Build history of the part. All positions in model axes, mm. A direction names the side the tool comes from. Give positions to 0.01 mm unless a question says otherwise; leave off trailing zeros. Loops run counter-clockwise (first coordinate to the right, second up) from the corner with the lowest first, then second, coordinate; pieces in that order, holes last. Notation, with made-up numbers: (-18, 38.25) -> (28, 38.25) arc R18 ccw to (28, 53.25) -> close; hole circle Ø1 at (43, -28.5). An arc over 180 degrees is marked (long way). Answer as a JSON object with one key per item and string values. Group by question number.
Q1. Band-saw the part on A-A, the plane x = 0. Write the cut outline in (y, z).
Q2. Band-saw the part on B-B, the plane y = 64.5. Write the cut outline in (x, z), plus the area to 3 significant figures.
Q3. Two-plate mould, pull along X, no slides. Class faces 4 (the flat face through (0, 96, -48.1)), 5 (the flat face through (-23, 0, 0)), 6 (the flat face through (21, 77.2, 5)): pulls with the +X half, pulls with the -X half, needs draft (parallel to the pull), parting line crosses it, or undercut.
Q4. Band-saw the part on C-C, the plane y = 0. Write the cut outline in (x, z), plus the area to 3 significant figures.
Q5. Tool access for faces 1 (the cylindrical face through (28.366, -3.312, -3.612)), 2 (the flat face through (28.762, 66, 4)), 3 (the flat face through (-6, 119.7, -2)): list every direction of +Z, -Z, +X, -X, +Y, -Y with a clear straight run to the whole face (end or side of a thin tool).
Q6. Band-saw the part on D-D, the plane z = -22.5. Write the cut outline in (x, y), plus the area to 3 significant figures.
Q7. Wall check: probe 1 along Y at (x, z) = (-15.5, -14); probe 2 along Y at (x, z) = (3, -12); probe 3 along Z at (x, y) = (4.5, 85.5). Give the ranges that are in metal, low to high. Write a range as from..to.
Q8. Drop flat-ended pins along their axis: pin 1 (17.5 mm diameter, centred on y = 27, z = 7, fed in from +X); pin 2 (1.4 mm diameter, centred on x = 27, y = 92.5, fed in from -Z); pin 3 (4 mm diameter, centred on x = 21.5, z = 10.5, fed in from +Y). Give the stop position or say it passes through.
from build123d import *

# Parameters (mm, degrees)
SKETCH1_W                 = 46
SKETCH1_H                 = 40.2
BOSS_EXTRUDE1_DEPTH       = 65.1
SKETCH3_R                 = 14
BOSS_EXTRUDE2_DEPTH       = 3
SKETCH4_R                 = 4.9
BOSS_EXTRUDE3_DEPTH       = 4.8
SKETCH7_W                 = 40.2
SKETCH7_H                 = 35.4
BOSS_EXTRUDE6_DEPTH       = 1
CHAMFER1_SIZE             = 6
CHAMFER1_SIZE2            = 5.1
MIRROR3_START             = 44.200099823
MIRROR3_OUTLINE_W         = 50
MIRROR3_OUTLINE_H         = 11
MIRROR3_DEPTH             = 3.885890521
CHAMFER1_OF_MIRROR8_SIZE2 = 5.1
CHAMFER1_OF_MIRROR8_SIZE  = 6
BOSS_EXTRUDE7_DEPTH       = 4.7625
SKETCH9_W                 = 40.2
SKETCH9_H                 = 61.1
BOSS_EXTRUDE8_DEPTH       = 41
SKETCH10_W                = 38
SKETCH10_H                = 38
BOSS_EXTRUDE9_DEPTH       = 9.3
SKETCH11_R                = 14
BOSS_EXTRUDE10_DEPTH      = 3
SKETCH12_R                = 4.9
BOSS_EXTRUDE11_DEPTH      = 4.8


# Read off the part's stored shape, not the designer's step: Mirror3
with BuildPart() as part:
    # Sketch1 → Boss-Extrude1 (new body)
    with BuildSketch(Plane(origin=(0, -14.5, 0), x_dir=(-1, 0, 0), z_dir=(0, 1, 0))):
        Rectangle(SKETCH1_W, SKETCH1_H)
    extrude(amount=BOSS_EXTRUDE1_DEPTH)

    # Sketch3 → Boss-Extrude2 (add)
    with BuildSketch(Plane.ZY.offset(-23)):
        Circle(SKETCH3_R)
    extrude(amount=-BOSS_EXTRUDE2_DEPTH)

    # Sketch4 → Boss-Extrude3 (add)
    with BuildSketch(Plane(origin=(26, 0, 0), x_dir=(0, 0, -1), z_dir=(1, 0, 0))):
        with Locations(Location((0, 0, 0), (0, 0, 180))):
            Circle(SKETCH4_R)
    extrude(amount=BOSS_EXTRUDE3_DEPTH)

    # Sketch7 → Boss-Extrude6 (add)
    with BuildSketch(Plane.ZY.offset(23)):
        with Locations((0, 32.9)):
            Rectangle(SKETCH7_W, SKETCH7_H)
    boss_extrude6 = extrude(amount=BOSS_EXTRUDE6_DEPTH)

    # Mirror1: Boss-Extrude6 across plane
    add(boss_extrude6.mirror(Plane(origin=(0, 0, 0), x_dir=(0, 0, 1), z_dir=(1, 0, 0))))

    # Chamfer1
    chamfer1_edges = [part.edges().sort_by_distance(p)[0] for p in [
        (0, 50.6, 20.1),
    ]]
    chamfer1_side = [part.faces().sort_by_distance(p)[0] for p in [
        (0, 18.392982971, 20.1),
    ]]
    chamfer(chamfer1_edges, length=CHAMFER1_SIZE, length2=CHAMFER1_SIZE2, reference=chamfer1_side[0])

    # Mirror3 outline → Mirror3 (cut)
    with BuildSketch(Plane(origin=(0, 0, 0), x_dir=(1, 0, 0), z_dir=(0, 0.6476484200955404, -0.7619393177594594)).offset(MIRROR3_START)):
        with Locations((0, -24.5)):
            Rectangle(MIRROR3_OUTLINE_W, MIRROR3_OUTLINE_H)
    mirror3 = extrude(amount=MIRROR3_DEPTH, mode=Mode.SUBTRACT)

    # Mirror8: Mirror3 across plane
    add(mirror3.mirror(Plane.ZX.offset(18.05)), mode=Mode.SUBTRACT)

    # Chamfer1 of Mirror8
    chamfer1_of_mirror8_edges = [part.edges().sort_by_distance(p)[0] for p in [
        (0, -14.5, 20.1),
    ]]
    chamfer(chamfer1_of_mirror8_edges, length=CHAMFER1_OF_MIRROR8_SIZE, length2=CHAMFER1_OF_MIRROR8_SIZE2)

    # Sketch8 → Boss-Extrude7 (add)
    with BuildSketch(Plane(origin=(24, 0, 0), x_dir=(0, 0, -1), z_dir=(1, 0, 0))):
        Polygon((20.1, 15.2), (8.9, 15.2), (-20.1, 31.2), (-20.1, 115.2), (8.9, 115.2), (8.9, 57.776470588), (20.1, 44.6), align=None)
    boss_extrude7 = extrude(amount=BOSS_EXTRUDE7_DEPTH)

    # Mirror4: Boss-Extrude7 across plane
    add(boss_extrude7.mirror(Plane(origin=(0, 0, 0), x_dir=(0, 0, 1), z_dir=(1, 0, 0))))



with BuildPart() as body_2:
    # Sketch9 → Boss-Extrude8 (new body)
    with BuildSketch(Plane(origin=(0, 116.7, 0), x_dir=(-1, 0, 0), z_dir=(0, 1, 0))):
        with Locations((0, -17.55)):
            Rectangle(SKETCH9_W, SKETCH9_H)
    extrude(amount=-BOSS_EXTRUDE8_DEPTH)


with BuildPart() as part_1:
    add(part.part)

    add(body_2.part)  # Boss-Extrude9 merges body 2
    # Sketch10 → Boss-Extrude9 (add)
    with BuildSketch(Plane.ZY.offset(-24)):
        with Locations((1.1, 96.2)):
            Rectangle(SKETCH10_W, SKETCH10_H)
    boss_extrude9 = extrude(amount=BOSS_EXTRUDE9_DEPTH)

    # Mirror6: Boss-Extrude9 across plane
    add(boss_extrude9.mirror(Plane(origin=(0, 0, 0), x_dir=(0, 0, 1), z_dir=(1, 0, 0))))

    # Sketch11 → Boss-Extrude10 (add)
    with BuildSketch(Plane(origin=(0, 116.7, 0), x_dir=(-1, 0, 0), z_dir=(0, 1, 0))):
        with Locations(Location((0, 0, 0), (0, 0, 68.213210702))):
            Circle(SKETCH11_R)
    extrude(amount=BOSS_EXTRUDE10_DEPTH)

    # Sketch12 → Boss-Extrude11 (add)
    with BuildSketch(Plane(origin=(0, 119.7, 0), x_dir=(1, 0, 0), z_dir=(0, 1, 0))):
        with Locations(Location((0, 0, 0), (0, 0, 270))):
            Circle(SKETCH12_R)
    extrude(amount=BOSS_EXTRUDE11_DEPTH)


solid = part_1.part
Worked answers:
{
 "1": {"outline": "(-14.5, -15) -> (-8.5, -20.1) -> (44.6, -20.1) -> (50.6, -15) -> (50.6, 15) -> (44.6, 20.1) -> (-8.5, 20.1) -> (-14.5, 15) -> close; (75.7, -48.1) -> (116.7, -48.1) -> (116.7, -14) -> (119.7, -14) -> (119.7, -4.9) -> (124.5, -4.9) -> (124.5, 4.9) -> (119.7, 4.9) -> (119.7, 14) -> (116.7, 14) -> (116.7, 13) -> (75.7, 13) -> close"},
 "2": {"outline": "(-28.76, -8.9) -> (-24, -8.9) -> (-24, 20.1) -> (-28.76, 20.1) -> close; (24, -8.9) -> (28.76, -8.9) -> (28.76, 20.1) -> (24, 20.1) -> close", "area": "276 mm2"},
 "3": {"face 4": "needs draft", "face 5": "pulls with the -X half", "face 6": "undercut"},
 "4": {"outline": "(-23, -20.1) -> (23, -20.1) -> (23, -14) -> (26, -14) -> (26, -4.9) -> (30.8, -4.9) -> (30.8, 4.9) -> (26, 4.9) -> (26, 14) -> (23, 14) -> (23, 20.1) -> (-23, 20.1) -> close", "area": "1,980 mm2"},
 "5": {"face 1": "+X", "face 2": "+Z, -Z, +X, +Y", "face 3": "+Y"},
 "6": {"outline": "(-20.1, 75.7) -> (20.1, 75.7) -> (20.1, 116.7) -> (-20.1, 116.7) -> close", "area": "1,650 mm2"},
 "7": {"probe 1": "-14.5..50.6, 75.7..116.7", "probe 2": "-14.5..50.6, 75.7..119.7", "probe 3": "-48.1..13"},
 "8": {"pin 1": "x = 28.76", "pin 2": "z = -8.9", "pin 3": "y = 116.7"}
}
